Source: three-view drawing plus pictorial views. Frame: mm from the lowest corner of the part. Coordinates: 2 decimals unless noted, no trailing zeros. Order: outer loops, then holes, each group sorted by start corner. A loop starts at its lowest first (then second) coordinate and runs counter-clockwise, first axis right, second up. Notation, with made-up numbers: (53, -38) -> (111, -38) arc R17 ccw to (111, -5) -> close; hole circle Ø9 at (32.25, 46). An arc over 180 degrees is marked (long way). Use one line per item in the form item = value. Start each with the question number.
1) Section query C-C on y = 31.5. Output: boundary loops of the cut face in (x, z).
2) Section query D-D on y = 11.5. Output: boundary loops of the cut face in (x, z).
3) Section query B-B on x = 16.5. Output: boundary loops of the cut face in (y, z).
4) Section query A-A on z = 0.5. Output: boundary loops of the cut face in (x, y).
5) Ray query, line 1 along Y through (x, z) = (16.5, 0.35); line 2 along X through (y, z) = (11, 0.8) (1 decimal); line 3 along X through (y, z) = (2.5, 0.45) (1 decimal). Return the intervals inside material, ascending.
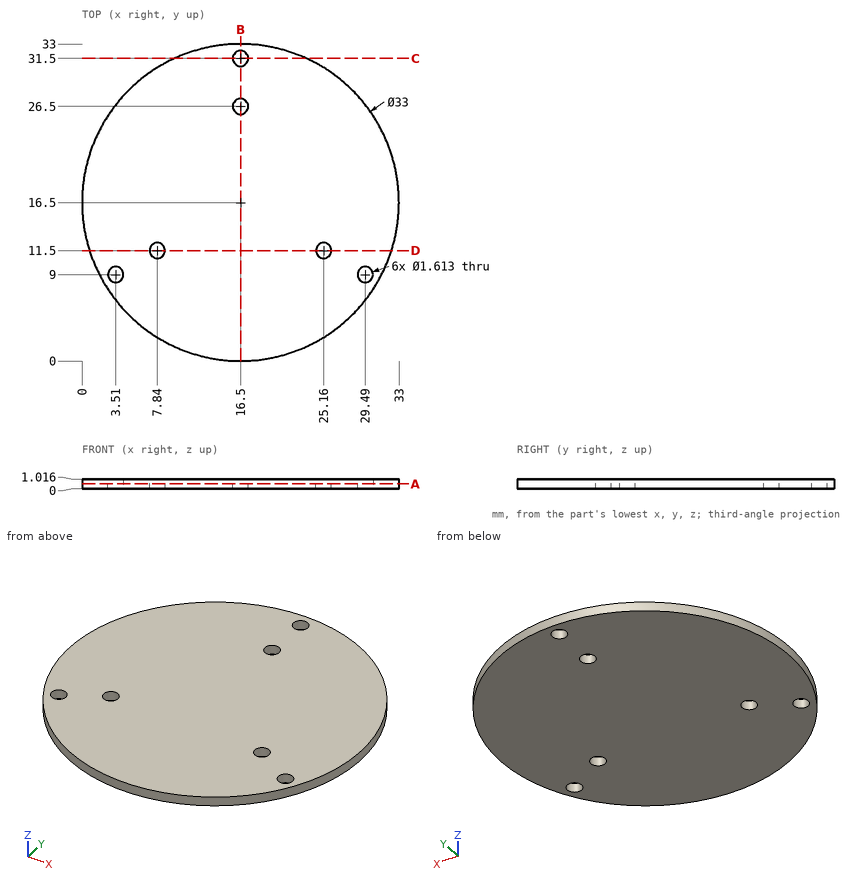
Answers below:
q1.outline = (9.63, 0) -> (15.69, 0) -> (15.69, 1.02) -> (9.63, 1.02) -> close; (17.31, 0) -> (23.37, 0) -> (23.37, 1.02) -> (17.31, 1.02) -> close
q2.outline = (0.78, 0) -> (7.03, 0) -> (7.03, 1.02) -> (0.78, 1.02) -> close; (8.65, 0) -> (24.35, 0) -> (24.35, 1.02) -> (8.65, 1.02) -> close; (25.97, 0) -> (32.22, 0) -> (32.22, 1.02) -> (25.97, 1.02) -> close
q3.outline = (0, 0) -> (25.69, 0) -> (25.69, 1.02) -> (0, 1.02) -> close; (27.31, 0) -> (30.69, 0) -> (30.69, 1.02) -> (27.31, 1.02) -> close; (32.31, 0) -> (33, 0) -> (33, 1.02) -> (32.31, 1.02) -> close
q4.outline = circle Ø33 at (16.5, 16.5); hole circle Ø1.61 at (3.51, 9); hole circle Ø1.61 at (7.84, 11.5); hole circle Ø1.61 at (16.5, 26.5); hole circle Ø1.61 at (16.5, 31.5); hole circle Ø1.61 at (25.16, 11.5); hole circle Ø1.61 at (29.49, 9)
q5.line_1 = 0 to 25.69, 27.31 to 30.69, 32.31 to 33
q5.line_2 = 0.9 to 7.2, 8.5 to 24.5, 25.8 to 32.1
q5.line_3 = 7.8 to 25.2
